Autodesk Inventor part; units mm, degrees
ref_plane "YZ Plane" through (0, 0, 0) normal (1, 0, 0) x (0, 1, 0)
ref_plane "XZ Plane" through (0, 0, 0) normal (0, 1, 0) x (-1, 0, 0)
ref_plane "XY Plane" through (0, 0, 0) normal (0, 0, 1) x (1, 0, 0)
sketch "Sketch1" plane through (0, 0, 0) normal (0, 1, 0) x (-1, 0, 0)
  line L0 (0, 0) -> (20, 0)
  line L1 (20, 0) -> (20, -40.5)
  line L2 (20, -40.5) -> (0, -40.5)
  line L3 (0, -40.5) -> (0, 0)
  dimension "d0" = 20
  dimension "d1" = 40.5
extrude "Extrusion1" add sketch "Sketch1" along normal blind 8.5
fillet "Fillet1" radius 4.25 4 edges at (-10, 8.5, 0) (-10, 0, 0) (-10, 8.5, -40.5) (-10, 0, -40.5)
chamfer "Chamfer1" distance 2 angle 45 8 edges at (0, 8.5, -20.25) (0, 7.2554, -39.2554) (0, 0, -20.25) (0, 7.2554, -1.2446) (-20, 8.5, -20.25) (-20, 7.2554, -1.2446) (-20, 0, -20.25) (-20, 7.2554, -39.2554)
equation "\"d4\" = 0.5 * d2"
properties part number "battery"
Source: CAD feature listing. Evaluate the final solid. Frame: model axes, mm. Round coordinates to 2 decimals unless told otherwise and drop trailing zeros. Loops run counter-clockwise (first coordinate to the right, second up) from the corner with the lowest first, then second, coordinate; pieces in that order, holes last.
1. Ray query, L1, parallel to Y at x = -0.75, z = -14.5; L2, parallel to Z at x = -9.75, y = 2; L3, parallel to Z at x = -6.25, y = 0.5. Return the intervals inside material, ascending.
2. Section query A-A on z = -6. Output: boundary loops of the cut face in (x, y), and give its area (3 significant figures).
3. Contact query for flat-ended pins moving along their axis: pin 1 (2 mm diameter, centred on x = -17.5, y = 2.5, fed in from +Z); pin 2 (1 mm diameter, centred on x = -2, y = 5.5, fed in from -Z). Output: stop coordinate, or through.
Answers below:
1. L1: y = 1.25 to 7.25
1. L2: z = -39.86 to -0.64
1. L3: z = -38.25 to -2.25
2. outline: (-20, 2) - (-18, 0) - (-2, 0) - (0, 2) - (0, 6.5) - (-2, 8.5) - (-18, 8.5) - (-20, 6.5) - close
2. area: 162 mm2
3. pin 1: stops at z = -0.07
3. pin 2: stops at z = -40.43
